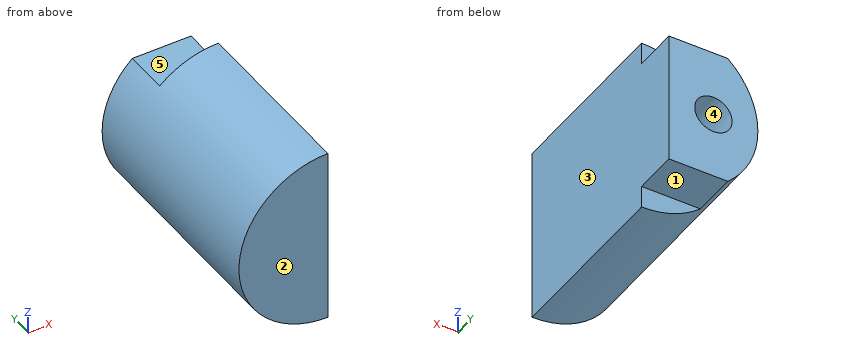
from build123d import *

# Parameters (mm, degrees)
BOSS_EXTRUDE1_DEPTH   = 25
CUT_EXTRUDE1_DEPTH    = 5
M5_TAPPED_HOLE1_D     = 4.2
M5_TAPPED_HOLE1_DEPTH = 11.1381927
M5_TAPPED_HOLE1_TIP   = 1.2618073


with BuildPart() as part:
    # Sketch1 → Boss-Extrude1 (new body)
    with BuildSketch(Plane(origin=(0, 0, 0), x_dir=(1, 0, 0), z_dir=(0, 1, 0))):
        with BuildLine():
            Line((0, 10), (0, -10))
            ThreePointArc((0, -10), (-10, 0), (0, 10))
        make_face()
    extrude(amount=BOSS_EXTRUDE1_DEPTH)

    # Sketch18 → Cut-Extrude1 (cut)
    with BuildSketch(Plane(origin=(0, 25, 0), x_dir=(1, 0, 0), z_dir=(0, 1, 0))):
        with BuildLine():
            Line((0, 7.5), (0, 10))
            ThreePointArc((0, 10), (-3.535533906, 9.354143467), (-6.614378278, 7.5))
            Line((-6.614378278, 7.5), (0, 7.5))
        make_face()
        with BuildLine():
            Line((0, -10), (0, -7.5))
            Line((0, -7.5), (-6.614378278, -7.5))
            ThreePointArc((-6.614378278, -7.5), (-3.535533906, -9.354143467), (0, -10))
        make_face()
    extrude(amount=-CUT_EXTRUDE1_DEPTH, mode=Mode.SUBTRACT)

    # M5 Tapped Hole1
    with Locations(Plane(origin=(0, 25, 0), x_dir=(1, 0, 0), z_dir=(0, 1, 0))):
        with Locations((-5, 0)):
            Hole(M5_TAPPED_HOLE1_D / 2, depth=M5_TAPPED_HOLE1_DEPTH)
            with Locations((0, 0, -(M5_TAPPED_HOLE1_DEPTH + M5_TAPPED_HOLE1_TIP / 2))):  # 118° drill point
                Cone(0, M5_TAPPED_HOLE1_D / 2, M5_TAPPED_HOLE1_TIP, mode=Mode.SUBTRACT)


solid = part.part
The listing builds one solid part. Answer for the finished solid, in the listing's coordinates (mm). Face numbers are marked on the shaded views. A direction names the side the tool comes from. Coordinates: 2 decimals unless noted, no trailing zeros. Write each loop counter-clockwise with the first axis right and the second up, starting at its lowest first coordinate (ties: lowest second). Pieces come first, ordered by that corner, then holes. Notation, with made-up numbers: M -29.5,73.5 L 2.5,73.5 A14 cw 2.5,86.5 Z; hole C 47.25,43 d7. An arc over 180 degrees is marked long. Put each result on its own line as item: value. Start each with the question number.
1. Consider line 1 (Z direction, x = -5, y = 20.5); line 2 (X direction, y = 6.75, z = -7.5); line 3 (Y direction, x = -3.25, z = 8.5). Determine where each line is inside the solid, lowest interval first. Write a range as from..to.
2. Which of the six approach directions +Z, -Z, +X, -X, +Y, -Y give full straight-line access (tool end or side, diameter ignored) to the marked faces 1 and 2?
3. Flat-ended cylindrical pins translate along their axes: P1, Ø1.5, axis at x = -2, y = 23, coming from the -Z side; P2, Ø3, axis at x = -3, y = 18, coming from the +Z side; P3, Ø0.8, axis at x = -3, z = 9, coming from the +Y side. Find the tip coordinate at first contact, or state that the pin passes through.
4. For a pull along X with two mould halves and no side action, classify the marked faces 3, 4 and 5 as pulls with the +X half, pulls with the -X half, needs draft (parallel to the pull), parting line crosses it, or undercut.
5. A cutting plane is placed at B-B on y = 5.75. Write down the section's boundary in (x, z).
6. A cutting plane is placed at C-C on x = -8. Write down the section's boundary in (y, z).
7. A cutting plane is placed at D-D on z = -6.75. Write down the section's boundary in (x, y), then the cut area to 3 significant figures.
8. A cutting plane is placed at A-A on y = 21.75. Write down the section's boundary in (x, z).
Resolved:
1. line 1: z = -7.5..-2.1, 2.1..7.5
1. line 2: x = -6.61..0
1. line 3: y = 0..20
2. face 1: -Z, +X, -X, +Y
2. face 2: +Z, -Z, +X, -X, -Y
3. P1: stops at z = -7.5
3. P2: stops at z = 9.89
3. P3: stops at y = 20
4. face 3: pulls with the +X half
4. face 4: undercut
4. face 5: needs draft
5. outline: M 0,-10 L 0,10 A10 ccw Z
6. outline: M 0,-6 L 25,-6 L 25,6 L 0,6 Z
7. outline: M -7.38,0 L 0,0 L 0,25 L -7.38,25 Z
7. area: 184 mm2
8. outline: M -6.61,-7.5 L 0,-7.5 L 0,7.5 L -6.61,7.5 A10 ccw Z; hole C -5,0 d4.2
